The listing builds one solid part. Answer for the finished solid, in the listing's coordinates (mm). A direction names the side the tool comes from. Round coordinates to 2 decimals unless told otherwise and drop trailing zeros. Write each loop counter-clockwise with the first axis right and the second up, starting at its lowest first coordinate (ties: lowest second). Pieces come first, ordered by that corner, then holes. Notation, with made-up numbers: (-12, 8) - (40, 8) arc R25 ccw to (40, 44) - close; hole circle Ø4 at (55, 89.5). An arc over 180 degrees is marked (long way). Answer in a Markdown table with one row per item.
from build123d import *

# Parameters (mm, degrees)
F1_DEPTH  = 104.14
F2_T      = -6.35
F4_D      = 3.81
F4_DEPTH  = 6.604
F4_TIP    = 1.1446394792
F6_DEPTH  = 12.7
F8_DEPTH  = 12.7
F9_R      = 6.35
F10_START = -6.35
F3_R      = 6.35
F10_DEPTH = 19.05
F12_DEPTH = 6.35
F13_D     = 6.5278
F13_DEPTH = 6.604
F13_TIP   = 1.9611489744


with BuildPart() as f1:
    # F0 (on Front) → F1 (new body)
    with BuildSketch(Plane.XZ):
        Polygon((-37.1921509504, 56.5943730235), (-39.7321509504, 56.5943730235), (-39.7321509504, -0.1851844968), (51.7078490496, -0.1851844968), (51.7078490496, 2.3548155032), align=None)
    extrude(amount=-F1_DEPTH)

    # F2 (hollow: no face is removed)
    offset(amount=F2_T, mode=Mode.SUBTRACT)

    # F4
    with Locations(Plane(origin=(15.0736214303, 0, 24.7060449314), x_dir=(0.8536585366, 0, -0.5208330855), z_dir=(0.5208330855, 0, 0.8536585366))):
        with Locations((-40.9056190746, 20.32), (-40.9056190746, 83.82), (22.5943809254, 83.82), (22.5943809254, 20.32)):
            Hole(F4_D / 2, depth=F4_DEPTH)
            with Locations((0, 0, -(F4_DEPTH + F4_TIP / 2))):  # 118° drill point
                Cone(0, F4_D / 2, F4_TIP, mode=Mode.SUBTRACT)

    # F5 (on face) → F6 (cut)
    with BuildSketch(Plane(origin=(15.0736214303, 0, 24.7060449314), x_dir=(0.8536585366, 0, -0.5208330855), z_dir=(0.5208330855, 0, 0.8536585366))):
        with BuildLine():
            ThreePointArc((-34.5556190746, 40.005), (-33.8116702988, 38.2089487758), (-32.0156190746, 37.465))
            Line((-32.0156190746, 37.465), (-18.0456190746, 37.465))
            ThreePointArc((-18.0456190746, 37.465), (-16.2495678504, 38.2089487758), (-15.5056190746, 40.005))
            Line((-15.5056190746, 40.005), (-15.5056190746, 64.135))
            ThreePointArc((-15.5056190746, 64.135), (-16.2495678504, 65.9310512242), (-18.0456190746, 66.675))
            Line((-18.0456190746, 66.675), (-32.0156190746, 66.675))
            ThreePointArc((-32.0156190746, 66.675), (-33.8116702988, 65.9310512242), (-34.5556190746, 64.135))
            Line((-34.5556190746, 64.135), (-34.5556190746, 40.005))
        make_face()
    extrude(amount=-F6_DEPTH, mode=Mode.SUBTRACT)

    # F7 (on face) → F8 (cut)
    with BuildSketch(Plane(origin=(-39.7321509504, 0, 0), x_dir=(0, -1, 0), z_dir=(-1, 0, 0))):
        with BuildLine():
            Line((-20.32, 41.3543730235), (-83.82, 41.3543730235))
            ThreePointArc((-83.82, 41.3543730235), (-88.3101280605, 39.494501084), (-90.17, 35.0043730235))
            Line((-90.17, 35.0043730235), (-90.17, 15.9543730235))
            ThreePointArc((-90.17, 15.9543730235), (-88.3101280605, 11.464244963), (-83.82, 9.6043730235))
            Line((-83.82, 9.6043730235), (-20.32, 9.6043730235))
            ThreePointArc((-20.32, 9.6043730235), (-15.8298719395, 11.464244963), (-13.97, 15.9543730235))
            Line((-13.97, 15.9543730235), (-13.97, 35.0043730235))
            ThreePointArc((-13.97, 35.0043730235), (-15.8298719395, 39.494501084), (-20.32, 41.3543730235))
        make_face()
    extrude(amount=-F8_DEPTH, mode=Mode.SUBTRACT)

    # F9
    f9_edges = [f1.edges().sort_by_distance(p)[0] for p in [
        (-0.055497, 6.35, 26.498032),
        (-0.055497, 97.79, 26.498032),
        (-33.382151, 6.35, 26.498032),
        (-33.382151, 97.79, 26.498032),
    ]]
    fillet(f9_edges, radius=F9_R)

    # F3 (on face) → F10 (cut)
    with BuildSketch(Plane(origin=(15.0736214303, 0, 24.7060449314), x_dir=(0.8536585366, 0, -0.5208330855), z_dir=(0.5208330855, 0, 0.8536585366)).offset(F10_START)):
        with Locations((22.5943809254, 83.82)):
            Circle(F3_R)
        with Locations((22.5943809254, 20.32)):
            Circle(F3_R)
    extrude(amount=-F10_DEPTH, mode=Mode.SUBTRACT)

    # F11 (on face) → F12 (cut)
    with BuildSketch(Plane(origin=(0, 0, -0.1851844968), x_dir=(1, 0, 0), z_dir=(0, 0, -1))):
        with BuildLine():
            ThreePointArc((-5.858374995, -42.1181075931), (-7.7182469345, -37.6279795325), (-12.208374995, -35.7681075931))
            Line((-12.208374995, -35.7681075931), (-18.558374995, -35.7681075931))
            ThreePointArc((-18.558374995, -35.7681075931), (-23.0485030555, -37.6279795325), (-24.908374995, -42.1181075931))
            Line((-24.908374995, -42.1181075931), (-24.908374995, -61.1681075931))
            ThreePointArc((-24.908374995, -61.1681075931), (-23.0485030555, -65.6582356536), (-18.558374995, -67.5181075931))
            Line((-18.558374995, -67.5181075931), (-12.208374995, -67.5181075931))
            ThreePointArc((-12.208374995, -67.5181075931), (-7.7182469345, -65.6582356536), (-5.858374995, -61.1681075931))
            Line((-5.858374995, -61.1681075931), (-5.858374995, -42.1181075931))
        make_face()
    extrude(amount=-F12_DEPTH, mode=Mode.SUBTRACT)

    # F13
    with Locations(Plane(origin=(0, 0, -0.1851844968), x_dir=(1, 0, 0), z_dir=(0, 0, -1))):
        with Locations((5.9878490496, -19.05), (5.9878490496, -85.09)):
            Hole(F13_D / 2, depth=F13_DEPTH)
            with Locations((0, 0, -(F13_DEPTH + F13_TIP / 2))):  # 118° drill point
                Cone(0, F13_D / 2, F13_TIP, mode=Mode.SUBTRACT)


solid = f1.part
(1) Section B-B (y = 94) is taken. Give the vertices of the cut face in (x, z), and give its area (3 significant figures).
Checked values:
| item | result |
|---|---|
| outline | (-39.73, -0.19) - (51.71, -0.19) - (51.71, 2.35) - (-37.19, 56.59) - (-39.73, 56.59) - close; hole (-32.84, 6.16) - (32.24, 6.16) - (-32.84, 45.87) - close |
| area | 1,490 mm2 |
(2) Flat-ended cylindrical pins translate along their axes: pin 1 (10 mm diameter, centred on x = 17.5, y = 68, fed in from +Z); pin 2 (10.5 mm diameter, centred on x = 5.99, y = 85.09, fed in from +Z); pin 3 (1 mm diameter, centred on y = 24.5, z = 19.5, fed in from -X). Find the tip coordinate at first contact, or state that the pin passes through.
Checked values:
| item | result |
|---|---|
| pin 1 | stops at z = 26.28 |
| pin 2 | stops at z = 33.45 |
| pin 3 | stops at x = 10.59 |
(3) Section A-A (y = 73) is taken. Give the vertices of the cut face in (x, z), and give its area (3 significant figures).
Checked values:
| item | result |
|---|---|
| outline | (-39.73, -0.19) - (51.71, -0.19) - (51.71, 2.35) - (-37.19, 56.59) - (-39.73, 56.59) - (-39.73, 41.35) - (-33.38, 41.35) - (-33.38, 46.83) - (33.27, 6.16) - (-33.38, 6.16) - (-33.38, 9.6) - (-39.73, 9.6) - close |
| area | 1,220 mm2 |
(4) For faces 1 (the flat face through (-16.056, 52.239, 40.031)), 2 (the flat face through (-15, 67.518, 3)), 3 (the cylindrical face through (-31.57, 8.26, 26.78)), 4 (the flat face through (-5.858, 52, 3)), determine the directions among +Z, -Z, +X, -X, +Y, -Y from which every point of the face is accessible in a straight line to the end or side of a thin tool.
Checked values:
| item | result |
|---|---|
| face 1 | -Z, +X |
| face 2 | -Z |
| face 3 | none |
| face 4 | +Z, -Z |
(5) For a pull along Y with two mould halves and no side action, classify faces 5 (the flat face through (-5, 0, 22)), 6 (the flat face through (-14, 97.79, 15)), 7 (the flat face through (51.708, 51, 1)) as pulls with the +Y half, pulls with the -Y half, needs draft (parallel to the pull), parting line crosses it, or undercut.
Checked values:
| item | result |
|---|---|
| face 5 | pulls with the -Y half |
| face 6 | undercut |
| face 7 | needs draft |
(6) Find the intervals of material crossed by line 1 (Y direction, x = 30, z = 6); line 2 (Y direction, x = -26, z = 12); line 3 (X direction, y = 19.05, z = 4), in increasing order.
Checked values:
| item | result |
|---|---|
| line 1 | y = 0 to 13.97, 26.67 to 77.47, 90.17 to 104.14 |
| line 2 | y = 0 to 6.35, 97.79 to 104.14 |
| line 3 | x = -39.73 to 2.72, 9.25 to 21.62, 36.2 to 49.01 |
